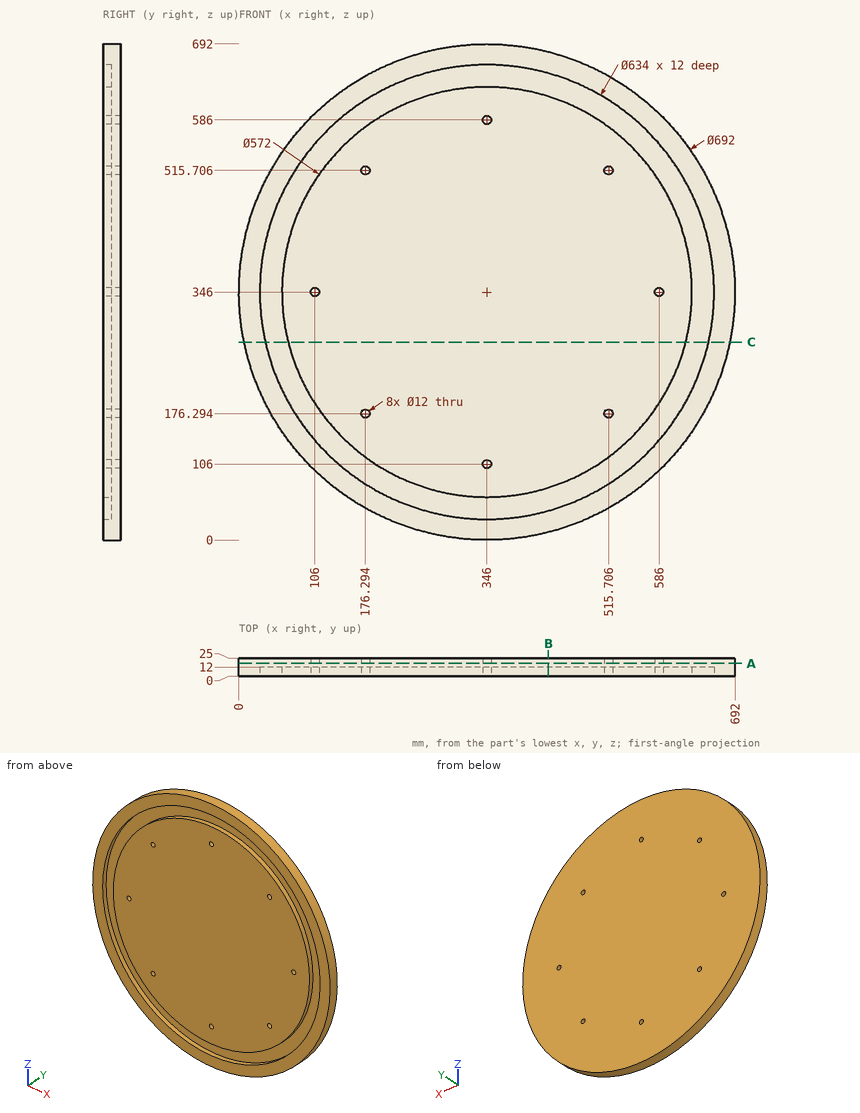
Input: dimensioned drawing with shaded views. Units: mm. Origin: part minimum x, y, z. Round coordinates to 2 decimals unless told otherwise and drop trailing zeros. Order: outer loops, then holes, each group sorted by start corner. A loop starts at its lowest first (then second) coordinate and runs counter-clockwise, first axis right, second up. Notation, with made-up numbers: (-31.5, 24.5) - (10.5, 24.5) arc R17 cw to (10.5, 34.5) - close; hole circle Ø8 at (-14, 40). An arc over 180 degrees is marked (long way). Write item = value, one per line. Start each with the question number.
Q1. Cut plane A-A on y = 17.75. Give the number of separate pieces and of enclosed holes in the cut face, and give its area (3 significant figures).
Q2. Cut plane C-C on z = 276. Return the cut outline in (x, y) (1 decimal), and give its area (3 significant figures).
Q3. Cut plane B-B on x = 431.5. Return the cut outline in (y, z).
Q4. Ray query, line 1 (X direction, y = 11.75, z = 346); line 2 (X direction, y = 8, z = 401); line 3 (X direction, y = 1.5, z = 432). Return the intervals inside material, ascending. Write a range as from..to.
Q5. Pin query (flat end, axial travel): pin 1 (10 mm diameter, centred on y = 15, z = 94, fed in from -X) (1 decimal); pin 2 (3 mm diameter, centred on x = 204.5, y = 20.5, fed in from -Z); pin 3 (6 mm diameter, centred on x = 446.5, y = 13, fed in from +Z). Return the tip coordinate at first contact, or that it passes through.
Outcome:
q1.separate_pieces = 1
q1.enclosed_holes = 8
q1.area = 375,000 mm^2
q2.outline = (7.2, 0) - (36.8, 0) - (36.8, 12) - (68.7, 12) - (68.7, 0) - (623.3, 0) - (623.3, 12) - (655.2, 12) - (655.2, 0) - (684.8, 0) - (684.8, 25) - (7.2, 25) - close
q2.area = 16,200 mm^2
q3.outline = (0, 10.73) - (25, 10.73) - (25, 681.27) - (0, 681.27) - (0, 651.25) - (12, 651.25) - (12, 618.92) - (0, 618.92) - (0, 73.08) - (12, 73.08) - (12, 40.75) - (0, 40.75) - close
q4.line_1 = 0..29, 60..100, 112..580, 592..632, 663..692
q4.line_2 = 4.4..33.81, 65.34..626.66, 658.19..687.6
q4.line_3 = 10.86..40.89, 73.24..618.76, 651.11..681.14
q5.pin_1 = 103.7
q5.pin_2 = 29.59
q5.pin_3 = 677.98
